Autodesk Inventor part; units mm, degrees
ref_plane "YZ Plane" through (0, 0, 0) normal (1, 0, 0) x (0, 1, 0)
ref_plane "XZ Plane" through (0, 0, 0) normal (0, 1, 0) x (-1, 0, 0)
ref_plane "XY Plane" through (0, 0, 0) normal (0, 0, 1) x (1, 0, 0)
sketch "Esboço1" plane through (0, 0, 0) normal (0, 1, 0) x (-1, 0, 0)
  circle A0 centre (0, 0) radius 2.1
  line L0 (0, 0) -> (0, 15)
  circle A1 centre (0, 15) radius 2
  line L1 (0, 0) -> (0, -15)
  circle A2 centre (0, -15) radius 2.1
  line L2 (0, 15) -> (-5.2, 15)
  line L3 (-5.2, 15) -> (-5.2, -15)
  line L4 (-5.2, -15) -> (0, -15)
  circle A3 centre (0, 0) radius 6.1
  circle A4 centre (0, 0) radius 24.7
  line L5 (0, 24.7) -> (24.7, 24.7)
  line L6 (24.7, 24.7) -> (24.7, 0)
  line L7 (24.7, 0) -> (0, 0)
  line L8 (0, 0) -> (0, 24.7)
  line L9 (24.7, 0) -> (0, 0)
  line L10 (0, 0) -> (0, -24.7)
  line L11 (0, -24.7) -> (24.7, -24.7)
  line L12 (24.7, -24.7) -> (24.7, 0)
  line L13 (0, -24.7) -> (-24.7, -24.7)
  line L14 (-24.7, -24.7) -> (-24.7, 0)
  line L15 (-24.7, 0) -> (0, 0)
  line L16 (0, 0) -> (0, -24.7)
  line L17 (0, 24.7) -> (-24.7, 24.7)
  line L18 (-24.7, 24.7) -> (-24.7, 0)
  line L19 (-24.7, 0) -> (0, 0)
  line L20 (0, 0) -> (0, 24.7)
  line L21 (-5.2, 15) -> (-5.2, 24.7)
  line L22 (-5.2, -15) -> (-5.2, -24.7)
  line L23 (-5.2, 24.7) -> (-24.7, 24.7)
  line L24 (-24.7, 24.7) -> (-24.7, -24.7)
  line L25 (-24.7, -24.7) -> (-5.2, -24.7)
  line L26 (-5.2, -24.7) -> (-5.2, 24.7)
  line L27 (0, -15) -> (0, -21.1)
  line L28 (0, -21.1) -> (-5.2, -21.1)
  line L29 (0, -15) -> (0, -8.9)
  line L30 (0, -8.9) -> (-5.2, -8.9)
  line L31 (0, -8.9) -> (0, -15)
  line L32 (0, 15) -> (0, 8.9)
  line L33 (0, 15) -> (0, 21.1)
  line L34 (0, 21.1) -> (-5.2, 21.1)
  line L35 (0, 8.9) -> (-5.2, 8.9)
  line L36 (6.1, 0) -> (6.1, -24.7)
  line L37 (6.1, 0) -> (6.1, 24.7)
  line L38 (-5.2, 21.1) -> (6.1, 21.1)
  line L39 (6.1, 21.1) -> (6.1, 24.7)
  line L40 (6.1, 24.7) -> (-5.2, 24.7)
  line L41 (-5.2, 24.7) -> (-5.2, 21.1)
  line L42 (-5.2, -21.1) -> (6.1, -21.1)
  line L43 (6.1, -21.1) -> (6.1, -24.7)
  line L44 (6.1, -24.7) -> (-5.2, -24.7)
  line L45 (-5.2, -24.7) -> (-5.2, -21.1)
  line L46 (6.1, 21.1) -> (0, 21.1)
  line L47 (0, 21.1) -> (0, 8.9)
  line L48 (0, 8.9) -> (6.1, 8.9)
  line L49 (6.1, 8.9) -> (6.1, 21.1)
  line L50 (0, -8.9) -> (6.1, -8.9)
  line L51 (6.1, -8.9) -> (6.1, -21.1)
  line L52 (6.1, -21.1) -> (0, -21.1)
  line L53 (0, -21.1) -> (0, -8.9)
  line L54 (6.1, -24.7) -> (9.1, -24.7)
  line L55 (9.1, -24.7) -> (9.1, 24.7)
  line L56 (9.1, 24.7) -> (6.1, 24.7)
  line L57 (6.1, 24.7) -> (6.1, -24.7)
  circle A5 centre (0, 0) radius 8.3
  circle A6 centre (0, 15) radius 8.3
  line L58 (-5.2, -8.9) -> (-24.7, -8.9)
  line L59 (-24.7, -8.9) -> (-24.7, -24.7)
  line L60 (-24.7, -24.7) -> (-5.2, -24.7)
  line L61 (-5.2, -24.7) -> (-5.2, -8.9)
  line L62 (-5.2, 8.9) -> (-24.7, 8.9)
  line L63 (-24.7, 8.9) -> (-24.7, 24.7)
  line L64 (-24.7, 24.7) -> (-5.2, 24.7)
  line L65 (-5.2, 24.7) -> (-5.2, 8.9)
  line L66 (-8.3, 0) -> (-8.3, -8.9)
  line L67 (-8.3, 0) -> (-8.3, 8.9)
  line L68 (-8.3, -8.9) -> (-8.8, -8.9)
  line L69 (-8.8, -8.9) -> (-8.8, 8.9)
  line L70 (-8.8, 8.9) -> (-8.3, 8.9)
  line L71 (-8.3, 8.9) -> (-8.3, -8.9)
  line L72 (-8.8, -8.9) -> (-24.7, -8.9)
  line L73 (-24.7, -8.9) -> (-24.7, -24.7)
  line L74 (-24.7, -24.7) -> (-8.8, -24.7)
  line L75 (-8.8, -24.7) -> (-8.8, -8.9)
  line L76 (-8.8, -8.9) -> (-24.7, -8.9)
  line L77 (-24.7, -8.9) -> (-24.7, 24.7)
  line L78 (-24.7, 24.7) -> (-8.8, 24.7)
  line L79 (-8.8, 24.7) -> (-8.8, -8.9)
  line L80 (9.1, -24.7) -> (6.1, -24.7)
  line L81 (6.1, -24.7) -> (6.1, -21.1)
  line L82 (6.1, -21.1) -> (9.1, -21.1)
  line L83 (9.1, -21.1) -> (9.1, -24.7)
  line L84 (6.1, 21.1) -> (9.1, 21.1)
  line L85 (9.1, 21.1) -> (9.1, 24.7)
  line L86 (9.1, 24.7) -> (6.1, 24.7)
  line L87 (6.1, 24.7) -> (6.1, 21.1)
  line L88 (9.1, 24.7) -> (9.1, 22.9)
  line L89 (-24.7, -24.7) -> (-21.7, -24.7)
  line L90 (-24.7, -21.1) -> (-24.7, -24.7)
  line L91 (-24.7, 24.7) -> (-21.7, 24.7)
  line L92 (-24.7, 21.1) -> (-24.7, 24.7)
  line L93 (-24.7, -24.7) -> (-20.2, -24.7)
  line L94 (-20.2, -24.7) -> (-20.2, -20.2)
  line L95 (-20.2, -20.2) -> (-24.7, -20.2)
  line L96 (-24.7, -20.2) -> (-24.7, -24.7)
  line L97 (-24.7, 24.7) -> (-20.2, 24.7)
  line L98 (-20.2, 24.7) -> (-20.2, 20.2)
  line L99 (-20.2, 20.2) -> (-24.7, 20.2)
  line L100 (-24.7, 20.2) -> (-24.7, 24.7)
  line L101 (-8.8, -24.7) -> (-13.3, -24.7)
  line L102 (-13.3, -24.7) -> (-13.3, -20.2)
  line L103 (-13.3, -20.2) -> (-8.8, -20.2)
  line L104 (-8.8, -20.2) -> (-8.8, -24.7)
  line L105 (-8.8, 24.7) -> (-13.3, 24.7)
  line L106 (-13.3, 24.7) -> (-13.3, 20.2)
  line L107 (-13.3, 20.2) -> (-8.8, 20.2)
  line L108 (-8.8, 20.2) -> (-8.8, 24.7)
  line L109 (-13.3, -22.45) -> (-8.8, -22.45)
  line L110 (-20.2, -22.45) -> (-24.7, -22.45)
  line L111 (-20.2, 22.45) -> (-24.7, 22.45)
  line L112 (-8.8, 22.45) -> (-13.3, 22.45)
  circle A7 centre (-11.05, -22.45) radius 1.55
  circle A8 centre (-22.45, -22.45) radius 1.55
  circle A9 centre (-11.05, 22.45) radius 1.55
  circle A10 centre (-22.45, 22.45) radius 1.55
  circle A11 centre (0, 0) radius 6.4
  point P0 (-5.2, -3.189)
  point P1 (-5.2, 3.189)
  point P2 (-5.2, 24.1464)
  point P3 (-5.2, -24.1464)
  point P4 (6.1, -21.1)
  point P5 (6.1, 21.1)
  dimension "d6" = 12.2
  dimension "d19" = 16.6
  dimension "d0" = 4.2
  dimension "d1" = 15
  dimension "d2" = 4
  dimension "d3" = 15
  dimension "d4" = 4.2
  dimension "d5" = 5.2
  dimension "d7" = 49.4
  dimension "d8" = 6.1
  dimension "d9" = 6.1
  dimension "d10" = 6.1
  dimension "d11" = 6.1
  dimension "d16" = 3
  dimension "d20" = 16.6
  dimension "d21" = 0.5
  dimension "d29" = 4.5
  dimension "d30" = 4.5
  dimension "d31" = 4.5
  dimension "d32" = 4.5
  dimension "d33" = 4.5
  dimension "d34" = 4.5
  dimension "d35" = 4.5
  dimension "d36" = 4.5
  dimension "d37" = 3.1
  dimension "d38" = 3.1
  dimension "d39" = 3.1
  dimension "d40" = 3.1
  dimension "d45" = 12.8
extrude "Extrusão1" add sketch "Esboço1" along normal blind 5 contours A3 L15 A11 L3 | L3 A11 L15 A3 | A11 L15 A5 L3 | L3 A5 L15 A11 | A5 L67 L62 A6 L3 | L3 L58 L66 A5 | L66 L58 L69 L15 | L15 L69 L62 L67 | A6 L62 L3 | L3 L22 A4 L75 L58 | L69 L58 A4 L15 | L15 A4 L62 L69 | L62 L79 A4 L21 A6 | L62 A6 L21 L3 | L75 L103 L102 A4 L58 | L62 A4 L106 L107 L79 | L75 L109 A7 A4 L102 L103 | L107 L106 A4 A9 L112 L79 | A4 A7 L109 L75 | L112 A9 A4 L79 | A4 L109 A7 | A4 L112 A9 | A7 L109 A4 | L112 A4 A9 picked at (-9.9489, -22.4881) picked at (-11.1489, 21.6171) picked at (-11.1489, -21.6171) picked at (-9.9489, 22.4881)
extrude "Extrusão2" add sketch "Esboço1" along normal blind 5 contours L36 A11 L1 A3 | A3 L0 A11 L37 | A3 L3 A11 L0 | L1 A11 L3 A3 | L36 A5 L1 A11 | A11 L0 A6 A5 L37 | A11 L3 A5 A6 L0 | L1 A5 L3 A11 | L36 L50 L1 A5 | A5 A6 L48 L37 | A6 A5 L0 | L0 A5 A6 | L1 L30 L3 A5 | A5 L0 L48 A6 | A5 A6 L3 L35 L0 | A5 L3 A6 | L36 A4 L10 L42 | L38 A6 L8 A4 L37 | L36 L11 A4 | L10 A4 L22 L28 | A4 L5 L37 | L38 L8 A6 | L13 L22 A4 | L18 L62 A4 | A4 L58 L14 | A6 L8 L34 L21 | L21 A4 L8 A6 | A4 L21 L17 | L22 L13 L75 A4 | L62 L18 L99 L98 L17 L106 A4 | A4 L102 L13 L94 L95 L14 L58 | A4 L79 L17 L21 | L75 L13 L102 L109 A7 A4 | L106 L112 A9 A4 | A4 A7 L109 L102 | L95 L94 L110 A8 L14 | L18 L111 A10 L98 L99 | A4 A9 L112 L106 L17 L79 | A7 L109 A4 | A9 L112 A4 | A4 L109 A7 | A4 L112 A9 | L13 L14 L110 A8 L94 | L18 L17 L98 L111 A10 | A8 L110 | L110 A8 | A10 L111 | L111 A10 picked at (-11.818, -22.5746) picked at (-11.7193, 22.131) picked at (-11.7193, -22.131) picked at (-11.818, 22.5746)
extrude "Extrusão3" add sketch "Esboço1" along normal blind 5 contours L37 A11 L7 | L7 A11 L36 | A11 L37 A5 L7 | L7 A5 L36 A11 | A5 L37 A6 L84 L55 L7 | L7 L55 L82 L36 A5 | L55 A4 L36 L82 | L84 L37 A4 L55 | L37 A6 | A4 L37 L5 L55 | L55 L11 L36 A4
extrude "Extrusão4" cut sketch "Esboço1" along normal through all contours A7 L109 A4 | A4 L109 A7 | A9 L112 A4 | A4 L112 A9 | A7 L109 A4 | A4 L109 A7 | L112 A4 A9 | A4 L112 A9 | A8 L110 | L110 A8 | A10 L111 | L111 A10
extrude "Extrusão5" add sketch "Esboço1" against normal blind 2.6 contours L36 A11 L1 A3 | L37 A11 L7 | L7 A11 L36 | A3 L0 A11 L37 | A3 L3 A11 L0 | L1 A11 L3 A3 | A11 L37 A5 L7 | L7 A5 L36 A11 | L36 A5 L1 A11 | A11 L0 A6 A5 L37 | A11 L3 A5 A6 L0 | A3 L15 A11 L3 | L1 A5 L3 A11 | L3 A11 L15 A3 | A5 L37 A6 L84 L55 L7 | L7 L55 L82 L36 A5 | L36 L50 L1 A5 | A5 A6 L48 L37 | A6 A5 L0 | L0 A5 A6 | A11 L15 A5 L3 | L1 L30 L3 A5 | L3 A5 L15 A11 | A5 L0 L48 A6 | A5 A6 L3 L35 L0 | A5 L3 A6 | A5 L67 L62 A6 L3 | L3 L58 L66 A5 | L55 A4 L36 L82 | L84 L37 A4 L55 | L36 A4 L10 L42 | L37 A6 | L66 L58 L69 L15 | L15 L69 L62 L67 | A6 L62 L3 | L3 L22 A4 L75 L58 | A4 L37 L5 L55 | L55 L11 L36 A4 | L38 A6 L8 A4 L37 | L36 L11 A4 | L10 A4 L22 L28 | L69 L58 A4 L15 | L15 A4 L62 L69 | L62 L79 A4 L21 A6 | L62 A6 L21 L3 | A4 L5 L37 | L38 L8 A6 | L13 L22 A4 | L18 L62 A4 | A4 L58 L14 | L75 L103 L102 A4 L58 | L62 A4 L106 L107 L79 | A6 L8 L34 L21 | L21 A4 L8 A6 | A4 L21 L17 | L22 L13 L75 A4 | L62 L18 L99 L98 L17 L106 A4 | A4 L102 L13 L94 L95 L14 L58 | L75 L109 A7 A4 L102 L103 | L107 L106 A4 A9 L112 L79 | A4 L79 L17 L21 | L75 L13 L102 L109 A7 A4 | A4 A7 L109 L75 | L106 L112 A9 A4 | A4 A7 L109 L102 | L95 L94 L110 A8 L14 | L18 L111 A10 L98 L99 | L112 A9 A4 L79 | A4 A9 L112 L106 L17 L79 | L13 L14 L110 A8 L94 | L18 L17 L98 L111 A10
extrude "Extrusão6" cut sketch "Esboço1" against normal blind 2.6 contours L7 L0 A0 | L7 A3 L1 A0 | A0 L0 A3 L7 | A0 L1 L7 | L0 L15 A0 | A0 L15 L3 A3 L0 | L1 A3 L3 L15 A0 | A0 L15 L1 | L36 A11 L1 A3 | L37 A11 L7 | L7 A11 L36 | A3 L0 A11 L37 | A3 L3 A11 L0 | L1 A11 L3 A3 | L15 A3 L3 | L3 A3 L15 | A3 L15 A11 L3 | L3 A11 L15 A3
extrude "Extrusão7" cut sketch "Esboço1" along normal through all contours L7 L0 A0 | L7 A3 L1 A0 | A0 L0 A3 L7 | A0 L1 L7 | L0 L15 A0 | A0 L15 L3 A3 L0 | L1 A3 L3 L15 A0 | A0 L15 L1 | L36 A11 L1 A3 | L37 A11 L7 | L7 A11 L36 | A3 L0 A11 L37 | A3 L3 A11 L0 | L1 A11 L3 A3 | L15 A3 L3 | L3 A3 L15 | A3 L15 A11 L3 | L3 A11 L15 A3
properties part number "peça1_3DPrint"
Geometry check sheet. Reference: the model listing, model coordinates, mm. A direction names the side the tool comes from. Coordinates: 2 decimals unless noted, no trailing zeros. Order: outer loops, then holes, each group sorted by start corner. A loop starts at its lowest first (then second) coordinate and runs counter-clockwise, first axis right, second up. Notation, with made-up numbers: (32, 61) - (72, 61) arc R19 ccw to (72, 84) - close; hole circle Ø11 at (36, 76). An arc over 180 degrees is marked (long way). Answer in a Markdown table with one row per item. Add a question column.
1. Material ranges on L1, parallel to X at y = 0.75, z = 22.45; L2, parallel to Z at x = 11.05, y = 0.75; L3, parallel to X at y = 1, z = -15, recorded low to high. Write a range as [from, to].
2. Section check D-D (x = 0). Enter the section's corners in (y, z).
3. Section check C-C (z = 0). Enter the section's corners in (x, y).
4. Section check A-A (z = -22.45). Enter the section's corners in (x, y).
5. Section check B-B (x = 22.45). Enter the section's corners in (y, z), plus the area to 3 significant figures.
6. Draft check along Z on faces 1 (the face through (24.7, 1, 0)), 2 (the face through (8, 1, 24.7)), 3 (the face through (-1, 1, 21.1)). Enter one of: +Z half, -Z half, draft (parallel to the pull), parting line (faces both ways), or undercut.
7. Access from +Z, -Z, +X, -X, +Y, -Y to the whole of each face (thin tool, end or side, straight path). Record for faces 4 (the face through (0, 1, -21.1)), 5 (the face through (-9.1, 1, 0)).
8. Gauge pin test, flat end, axial feed: pin 1 Ø14.5 at (x, z) = (0, 0) entering from -Y. Record the tip position at first contact, or that the pin passes through.
Data:
| question | item | result |
|---|---|---|
| 1 | L1 | x = [-9.1, 9.5], [12.6, 20.9], [24, 24.7] |
| 1 | L2 | z = [-24.7, -24], [-20.9, 20.9], [24, 24.7] |
| 1 | L3 | x = [-9.1, -6.1], [5.2, 24.7] |
| 2 | outline | (-2.6, -24.7) - (5, -24.7) - (5, -21.1) - (-2.6, -21.1) - close; (-2.6, -8.9) - (5, -8.9) - (5, -6.4) - (-2.6, -6.4) - close; (-2.6, 6.4) - (5, 6.4) - (5, 8.9) - (-2.6, 8.9) - close; (-2.6, 21.1) - (5, 21.1) - (5, 24.7) - (-2.6, 24.7) - close |
| 3 | outline | (-9.1, -2.6) - (-6.4, -2.6) - (-6.4, 5) - (-9.1, 5) - close; (6.4, -2.6) - (24.7, -2.6) - (24.7, 5) - (6.4, 5) - close |
| 4 | outline | (-9.1, -2.6) - (9.5, -2.6) - (9.5, 5) - (-9.1, 5) - close; (12.6, -2.6) - (20.9, -2.6) - (20.9, 5) - (12.6, 5) - close; (24, -2.6) - (24.7, -2.6) - (24.7, 5) - (24, 5) - close |
| 5 | outline | (-2.6, -24.7) - (5, -24.7) - (5, -24) - (-2.6, -24) - close; (-2.6, -20.9) - (5, -20.9) - (5, 20.9) - (-2.6, 20.9) - close; (-2.6, 24) - (5, 24) - (5, 24.7) - (-2.6, 24.7) - close |
| 5 | area | 328 mm² |
| 6 | face 1 | draft |
| 6 | face 2 | +Z half |
| 6 | face 3 | undercut |
| 7 | face 4 | +Y, -Y |
| 7 | face 5 | +Z, -Z, -X, +Y, -Y |
| 8 | pin 1 | stops at y = -2.6 |
